```python
from build123d import *

# Parameters (mm, degrees)
SKETCH1_W               = 100
SKETCH1_H               = 64
BOSS_EXTRUDE1_DEPTH     = 12
CUT_EXTRUDE1_DEPTH      = 61.564015719
CUT_EXTRUDE1_DEPTH_BACK = 61.564015719
SKETCH2_R               = 12
SKETCH3_W               = 12
SKETCH3_H               = 40
BOSS_EXTRUDE2_DEPTH     = 46
SKETCH4_R               = 10
BOSS_EXTRUDE3_DEPTH     = 12
FILLET1_R               = 12


with BuildPart() as part:
    # Sketch1 → Boss-Extrude1 (new body)
    with BuildSketch(Plane(origin=(0, 0, 0), x_dir=(1, 0, 0), z_dir=(0, 1, 0))):
        Rectangle(SKETCH1_W, SKETCH1_H)
    extrude(amount=BOSS_EXTRUDE1_DEPTH)

    # Sketch2 → Cut-Extrude1 (cut, two sides: drawn at the far end of the back side and taken through both)
    with BuildSketch(Plane(origin=(0, 12, 0), x_dir=(1, 0, 0), z_dir=(0, 1, 0)).offset(-CUT_EXTRUDE1_DEPTH_BACK)):
        with Locations(Location((0, 0, 0), (0, 0, 270))):
            Circle(SKETCH2_R)
        with Locations(Location((30, 0, 0), (0, 0, 270))):
            Circle(SKETCH2_R)
    extrude(amount=CUT_EXTRUDE1_DEPTH + CUT_EXTRUDE1_DEPTH_BACK, mode=Mode.SUBTRACT)

    # Sketch3 → Boss-Extrude2 (add)
    with BuildSketch(Plane(origin=(0, 12, 0), x_dir=(1, 0, 0), z_dir=(0, 1, 0))):
        with Locations((-44, 0)):
            Rectangle(SKETCH3_W, SKETCH3_H)
    extrude(amount=BOSS_EXTRUDE2_DEPTH)

    # Sketch4 → Boss-Extrude3 (add)
    with BuildSketch(Plane(origin=(0, 58, 0), x_dir=(1, 0, 0), z_dir=(0, 1, 0))):
        with BuildLine():
            Line((-50, 20), (-70, 20))
            ThreePointArc((-70, 20), (-90, 0), (-70, -20))
            Line((-70, -20), (-50, -20))
            Line((-50, -20), (-38, -20))
            Line((-38, -20), (-38, 20))
            Line((-38, 20), (-50, 20))
        make_face()
        with Locations(Location((-70, 0, 0), (0, 0, 270))):
            Circle(SKETCH4_R, mode=Mode.SUBTRACT)
    extrude(amount=BOSS_EXTRUDE3_DEPTH)

    # Fillet1
    fillet1_edges = [part.edges().sort_by_distance(p)[0] for p in [
        (-44, 12, -20),
        (-44, 12, 20),
    ]]
    fillet(fillet1_edges, radius=FILLET1_R - 0.0001)  # a hair under: the kernel refuses the full size


solid = part.part
```
CAD build for the part. Positions are in the model's coordinates, mm. A direction names the side the tool comes from. Round coordinates to 2 decimals unless told otherwise and drop trailing zeros. Loops run counter-clockwise (first coordinate to the right, second up) from the corner with the lowest first, then second, coordinate; pieces in that order, holes last. Notation, with made-up numbers: M 56,62 L 96,62 A15 ccw 96,78 Z; hole C 64,51.5 d3. An arc over 180 degrees is marked long. Return JSON: item names as keys, results as strings. Group by question number.
(1) Saw through at D-D, the plane y = 15.5. List the corners of the cut face in (x, z), and give its area (3 significant figures).
(2) Saw through at A-A, the plane x = 30. List the corners of the cut face in (y, z), and give its area (3 significant figures).
(3) Saw through at B-B, the plane z = 0. List the corners of the cut face in (x, y), and give its area (3 significant figures).
(4) Saw through at C-C, the plane y = 43.5. List the corners of the cut face in (x, z), and give its area (3 significant figures).
(5) Mould opens along X. For faces 1 (the cylindrical face through (3.604, 5.916, 11.446)), 2 (the cylindrical face through (33.604, 5.916, 11.446)), 3 (the cylindrical face through (-90, 64, 0)), 4 (the flat face through (-12, 0, -8)) say: +X half, -X half, draft (parallel to the pull), parting line (faces both ways), or undercut.
(6) Tool access for faces 5 (the flat face through (-57, 58, 0)), 6 (the flat face through (10, 12, -8)), 7 (the flat face through (-47, 52, -20)), 8 (the flat face through (-47, 52, 20)): list every direction of +Z, -Z, +X, -X, +Y, -Y with a clear straight run to the whole face (end or side of a thin tool).
(7) Wall check: probe 1 along X at (y, z) = (5, 0); probe 2 along X at (y, z) = (65, 0); probe 3 along Z at (x, y) = (30, 7). Give the ranges that are in metal, low to high. Write a range as [from, to].
(8) Drop flat-ended pins along their axis: P1, Ø1, axis at x = 35.5, z = -15, coming from the +Y side; P2, Ø5, axis at y = 14, z = 4, coming from the +X side; P3, Ø9.5, axis at x = -48, y = 46.5, coming from the -Z side; P4, Ø17.5, axis at y = 39, z = -16, coming from the +X side. Give the stop position or say it passes through.
Answer list:
{
 "1": {"outline": "M -50,-23.53 L -38,-23.53 L -38,23.53 L -50,23.53 Z", "area": "565 mm2"},
 "2": {"outline": "M 0,-32 L 12,-32 L 12,-12 L 0,-12 Z; M 0,12 L 12,12 L 12,32 L 0,32 Z", "area": "480 mm2"},
 "3": {"outline": "M -90,58 L -80,58 L -80,70 L -90,70 Z; M -60,58 L -50,58 L -50,0 L -12,0 L -12,12 L -38,12 L -38,70 L -60,70 Z; M 12,0 L 18,0 L 18,12 L 12,12 Z; M 42,0 L 50,0 L 50,12 L 42,12 Z", "area": "1,560 mm2"},
 "4": {"outline": "M -50,-20 L -38,-20 L -38,20 L -50,20 Z", "area": "480 mm2"},
 "5": {"face 1": "undercut", "face 2": "undercut", "face 3": "-X half", "face 4": "draft"},
 "6": {"face 5": "+Z, -Z, -X, -Y", "face 6": "+Z, -Z, +X, +Y", "face 7": "-Z, +X, -X, +Y", "face 8": "+Z, +X, -X, +Y"},
 "7": {"probe 1": "[-50, -12], [12, 18], [42, 50]", "probe 2": "[-90, -80], [-60, -38]", "probe 3": "[-32, -12], [12, 32]"},
 "8": {"P1": "y = 12", "P2": "x = 50", "P3": "z = -20", "P4": "x = -38"}
}
